Work out the finished part from the listing and answer in its coordinate system (mm). Face numbers are marked on the shaded views. A direction names the side the tool comes from. Round coordinates to 2 decimals unless told otherwise and drop trailing zeros. Loops run counter-clockwise (first coordinate to the right, second up) from the corner with the lowest first, then second, coordinate; pieces in that order, holes last. Notation, with made-up numbers: (40, -19.5) - (70, -19.5) arc R23 ccw to (70, 8.5) - close; hole circle Ø7 at (38, 84.5). An arc over 180 degrees is marked (long way). Return JSON: item names as keys, results as strings.
from build123d import *

# Parameters (mm, degrees)
BOSS_EXTRUDE1_DEPTH            = 38.1
FILLET1_R                      = 2.54
CUT_EXTRUDE1_DEPTH             = 2.54
F_6_0_204_DIAMETER_HOLE1_D     = 5.1816
F_6_0_204_DIAMETER_HOLE1_DEPTH = 12.7
F_6_0_204_DIAMETER_HOLE1_TIP   = 1.556709692
CUT_EXTRUDE2_DEPTH             = 2.54
F_6_0_204_DIAMETER_HOLE2_D     = 5.1816
F_6_0_204_DIAMETER_HOLE2_DEPTH = 12.7
F_6_0_204_DIAMETER_HOLE2_TIP   = 1.556709692


with BuildPart() as part:
    # Sketch1 → Boss-Extrude1 (new body)
    with BuildSketch(Plane.XY):
        with BuildLine():
            ThreePointArc((-73.049046132, 12.7), (-31.115, 43.815), (10.819046132, 12.7))
            Line((10.819046132, 12.7), (63.1825, 12.7))
            Line((63.1825, 12.7), (63.1825, 50.8))
            Line((63.1825, 50.8), (75.8825, 50.8))
            Line((75.8825, 50.8), (75.8825, 0))
            Line((75.8825, 0), (0, 0))
            ThreePointArc((0, 0), (-31.115, 31.115), (-62.23, 0))
            Line((-62.23, 0), (-92.099046132, 0))
            Line((-92.099046132, 0), (-92.099046132, 12.7))
            Line((-92.099046132, 12.7), (-73.049046132, 12.7))
        make_face()
    extrude(amount=BOSS_EXTRUDE1_DEPTH)

    # Fillet1
    fillet1_edges = [part.edges().sort_by_distance(p)[0] for p in [
        (10.819046132, 12.7, 19.05),
        (63.1825, 50.8, 19.05),
        (75.8825, 50.8, 19.05),
        (75.8825, 0, 19.05),
        (0, 0, 19.05),
        (-62.23, 0, 19.05),
        (-92.099046132, 0, 19.05),
        (-92.099046132, 12.7, 19.05),
        (-73.049046132, 12.7, 19.05),
    ]]
    fillet(fillet1_edges, radius=FILLET1_R)

    # Sketch3 → Cut-Extrude1 (cut)
    with BuildSketch(Plane(origin=(0, 12.7, 0), x_dir=(1, 0, 0), z_dir=(0, 1, 0))):
        Polygon((33.325436464, -16.395689872), (33.325436464, -21.704310128), (37.922836464, -24.358620255), (42.520236464, -21.704310128), (42.520236464, -16.395689872), (37.922836464, -13.741379745), align=None)
        Polygon((-82.22610953, -13.741379745), (-86.82350953, -16.395689872), (-86.82350953, -21.704310128), (-82.22610953, -24.358620255), (-77.62870953, -21.704310128), (-77.62870953, -16.395689872), align=None)
    extrude(amount=-CUT_EXTRUDE1_DEPTH, mode=Mode.SUBTRACT)

    # #6 (0.204) Diameter Hole1
    with Locations(Plane(origin=(0, 12.7, 0), x_dir=(1, 0, 0), z_dir=(0, 1, 0))):
        with Locations((-82.22610953, -19.05), (37.922836464, -19.05)):
            Hole(F_6_0_204_DIAMETER_HOLE1_D / 2, depth=F_6_0_204_DIAMETER_HOLE1_DEPTH)
            with Locations((0, 0, -(F_6_0_204_DIAMETER_HOLE1_DEPTH + F_6_0_204_DIAMETER_HOLE1_TIP / 2))):  # 118° drill point
                Cone(0, F_6_0_204_DIAMETER_HOLE1_D / 2, F_6_0_204_DIAMETER_HOLE1_TIP, mode=Mode.SUBTRACT)

    # Sketch6 → Cut-Extrude2 (cut)
    with BuildSketch(Plane.ZY.offset(-63.1825)):
        Polygon((12.350437166, 28.070765011), (12.071677287, 33.372061262), (7.341240122, 35.781296251), (2.889562834, 32.889234989), (3.168322713, 27.587938738), (7.898759878, 25.178703749), align=None)
        Polygon((35.210437166, 28.070765011), (34.931677287, 33.372061262), (30.201240122, 35.781296251), (25.749562834, 32.889234989), (26.028322713, 27.587938738), (30.758759878, 25.178703749), align=None)
    extrude(amount=-CUT_EXTRUDE2_DEPTH, mode=Mode.SUBTRACT)

    # #6 (0.204) Diameter Hole2
    with Locations(Plane.ZY.offset(-65.7225)):
        with Locations((30.48, 30.48), (7.62, 30.48)):
            Hole(F_6_0_204_DIAMETER_HOLE2_D / 2, depth=F_6_0_204_DIAMETER_HOLE2_DEPTH)
            with Locations((0, 0, -(F_6_0_204_DIAMETER_HOLE2_DEPTH + F_6_0_204_DIAMETER_HOLE2_TIP / 2))):  # 118° drill point
                Cone(0, F_6_0_204_DIAMETER_HOLE2_D / 2, F_6_0_204_DIAMETER_HOLE2_TIP, mode=Mode.SUBTRACT)


solid = part.part
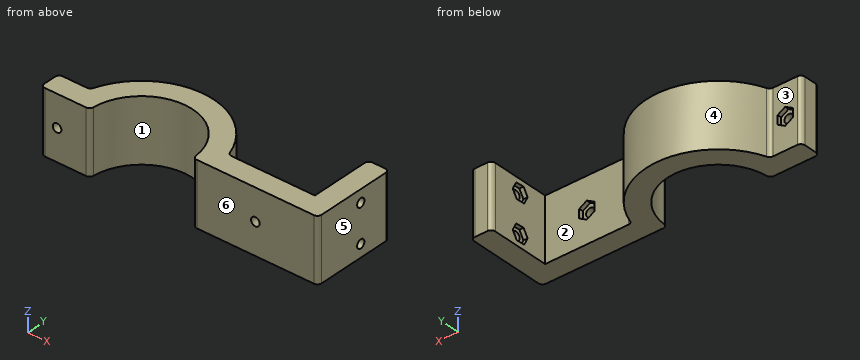
1) Flat-ended cylindrical pins translate along their axes: pin 1 (8.5 mm diameter, centred on y = 30.48, z = 30.48, fed in from -X); pin 2 (6 mm diameter, centred on x = 37.92, z = 19.05, fed in from -Y); pin 3 (3 mm diameter, centred on y = 35, z = 29.5, fed in from -X); pin 4 (10 mm diameter, centred on x = 37, z = 17.5, fed in from +Y). Find the tip coordinate at first contact, or state that the pin passes through.
Verdict:
{"pin 1": "stops at x = -66.21", "pin 2": "stops at y = 0", "pin 3": "stops at x = -59.36", "pin 4": "stops at y = 12.7"}
2) Find the intervals of material crossed by L1, parallel to X at y = 3.25, z = 19.05; L2, parallel to Y at x = 72.25, z = 7.62; L3, parallel to X at y = 15.5, z = 9, in increasing order.
Verdict:
{"L1": "x = -92.1 to -84.82, -79.64 to -62.06, -0.17 to 35.33, 40.51 to 75.88", "L2": "y = 0 to 27.89, 33.07 to 50.8", "L3": "x = -72.1 to -58.09, -4.14 to 9.87, 63.18 to 75.88"}
3) Section C-C (x = 54) is taken. Give the vertices of the cut face in (y, z), and give its area (3 significant figures).
Verdict:
{"outline": "(0, 0) - (12.7, 0) - (12.7, 38.1) - (0, 38.1) - close", "area": "484 mm2"}
4) A tool of negligible diameter and unlimited length cuts with its end or side. For the marked faces 1, 2 and 3, from which of +Z, -Z, +X, -X, +Y, -Y can it reach the whole face along a straight path? Write none if from no direction.
Verdict:
{"face 1": "+Z, -Z, -Y", "face 2": "+Z, -Z, +Y", "face 3": "+Z, -Z, -X, +Y"}
5) Section A-A (y = 23) is taken. Give the vertices of the cut face in (x, z).
Verdict:
{"outline": "(-68.41, 0) - (-52.07, 0) - (-52.07, 38.1) - (-68.41, 38.1) - close; (-10.16, 0) - (6.18, 0) - (6.18, 38.1) - (-10.16, 38.1) - close; (63.18, 0) - (75.88, 0) - (75.88, 38.1) - (63.18, 38.1) - close"}
6) Section D-D (x = -66.5) is taken. Give the vertices of the cut face in (y, z).
Verdict:
{"outline": "(0, 0) - (25.84, 0) - (25.84, 38.1) - (0, 38.1) - close"}
7) Section B-B (z = 19.05) is taken. Count the separate pieces of the cut face and the enclosed holes in it, and give its area (3 significant figures).
Verdict:
{"separate pieces": "3", "enclosed holes": "0", "area": "2,850 mm2"}
8) Determine the mould class of the marked faces 4, 5 and 6 for opening direction X: pulls with the +X half, pulls with the -X half, needs draft (parallel to the pull), parting line crosses it, or undercut.
Verdict:
{"face 4": "undercut", "face 5": "pulls with the +X half", "face 6": "needs draft"}
